```python
from build123d import *

# Parameters (mm, degrees)
CROQUIS1_W              = 28.5
CROQUIS1_H              = 125
SALIENTE_EXTRUIR1_DEPTH = 6
CROQUIS2_W              = 4.5
CROQUIS2_H              = 125
SALIENTE_EXTRUIR2_DEPTH = 5
CROQUIS3_R              = 6
CORTAR_EXTRUIR1_DEPTH   = 7


with BuildPart() as part:
    # Croquis1 → Saliente-Extruir1 (new body)
    with BuildSketch(Plane.XY):
        with Locations((14.25, 62.5)):
            Rectangle(CROQUIS1_W, CROQUIS1_H)
    extrude(amount=SALIENTE_EXTRUIR1_DEPTH)

    # Croquis2 → Saliente-Extruir2 (add)
    with BuildSketch(Plane.XY.offset(6)):
        with Locations((2.25, 62.5)):
            Rectangle(CROQUIS2_W, CROQUIS2_H)
    extrude(amount=SALIENTE_EXTRUIR2_DEPTH)

    # Croquis3 → Cortar-Extruir1 (cut, through all)
    with BuildSketch(Plane.XY.offset(6)):
        with Locations((28.5, 125)):
            Circle(CROQUIS3_R)
    extrude(amount=-CORTAR_EXTRUIR1_DEPTH, mode=Mode.SUBTRACT)


solid = part.part
```
Read the model definition and answer for the solid it produces. Units are mm, in the model's axes. A direction names the side the tool comes from. Coordinates: 2 decimals unless noted, no trailing zeros. Loops run counter-clockwise (first coordinate to the right, second up) from the corner with the lowest first, then second, coordinate; pieces in that order, holes last.
(1) Consider line 1 along X through (y, z) = (50, 6.25); line 2 along Z through (x, y) = (18.75, 24). Determine where each line is inside the solid, lowest interval first.
Solution:
line 1: x = 0 to 4.5
line 2: z = 0 to 6
(2) The part is cut by section B-B (y = 61). Determine the outline of the cut face in (x, z).
Solution:
outline: (0, 0) - (28.5, 0) - (28.5, 6) - (4.5, 6) - (4.5, 11) - (0, 11) - close
(3) A tool of negligible diameter and unlimited length cuts with its end or side. For faces 1 (the face through (2, 63, 11)), 2 (the face through (4.5, 62, 8)), from which of +Z, -Z, +X, -X, +Y, -Y can it reach the whole face along a straight path? Write none if from no direction.
Solution:
face 1: +Z, +X, -X, +Y, -Y
face 2: +Z, +X, +Y, -Y
(4) The part is cut by section C-C (z = 9.25). Determine the outline of the cut face in (x, y), and give its area (4 significant figures).
Solution:
outline: (0, 0) - (4.5, 0) - (4.5, 125) - (0, 125) - close
area: 562.5 mm2
(5) The part is cut by section A-A (x = 14.25). Determine the outline of the cut face in (y, z), and give its area (3 significant figures).
Solution:
outline: (0, 0) - (125, 0) - (125, 6) - (0, 6) - close
area: 750 mm2
(6) Flat-ended cylindrical pins translate along their axes: pin 1 Ø3 at (x, y) = (10.5, 69.5) entering from +Z; pin 2 Ø2.5 at (y, z) = (33.5, 9.5) entering from +X. Find the tip coordinate at first contact, or state that the pin passes through.
Solution:
pin 1: stops at z = 6
pin 2: stops at x = 4.5
